Geometry: see drawing. Coordinates: mm, zero at the bounding-box minimum. A direction names the side the tool comes from. Coordinates: 2 decimals unless noted, no trailing zeros. Write each loop counter-clockwise with the first axis right and the second up, starting at its lowest first coordinate (ties: lowest second). Pieces come first, ordered by that corner, then holes.
1) Section query A-A (x = 18.85). Output: boundary loops of the cut face in (y, z), then the cut area to 3 significant figures.
2) Section query D-D (z = 5). Output: boundary loops of the cut face in (x, y).
3) Set-up query: the marked faces 1 and 2. Return all of +Z, -Z, +X, -X, +Y, -Y with unobstructed straight access to the full face (end or side cutting, diameter ignored); none if empty.
4) Section query B-B (z = 24.09). Output: boundary loops of the cut face in (x, y), then the cut area to 3 significant figures.
5) Section query C-C (x = 29.85). Output: boundary loops of the cut face in (y, z).
6) Line query: L1, parallel to Y at x = 5, z = 24.09; L2, parallel to Y at x = 29.85, z = 8.3; L3, parallel to Y at x = 40.85, z = 5.5. Output: solid intervals per line, ascending.
7) Pin query (flat end, axial travel): pin 1 Ø4 at (y, z) = (10, 49.09) entering from +X; pin 2 Ø16.5 at (x, y) = (29.85, 20) entering from +Z; pin 3 Ø1 at (x, y) = (43.5, 29.5) entering from +Z. Return the tip coordinate at first contact, or that it passes through.
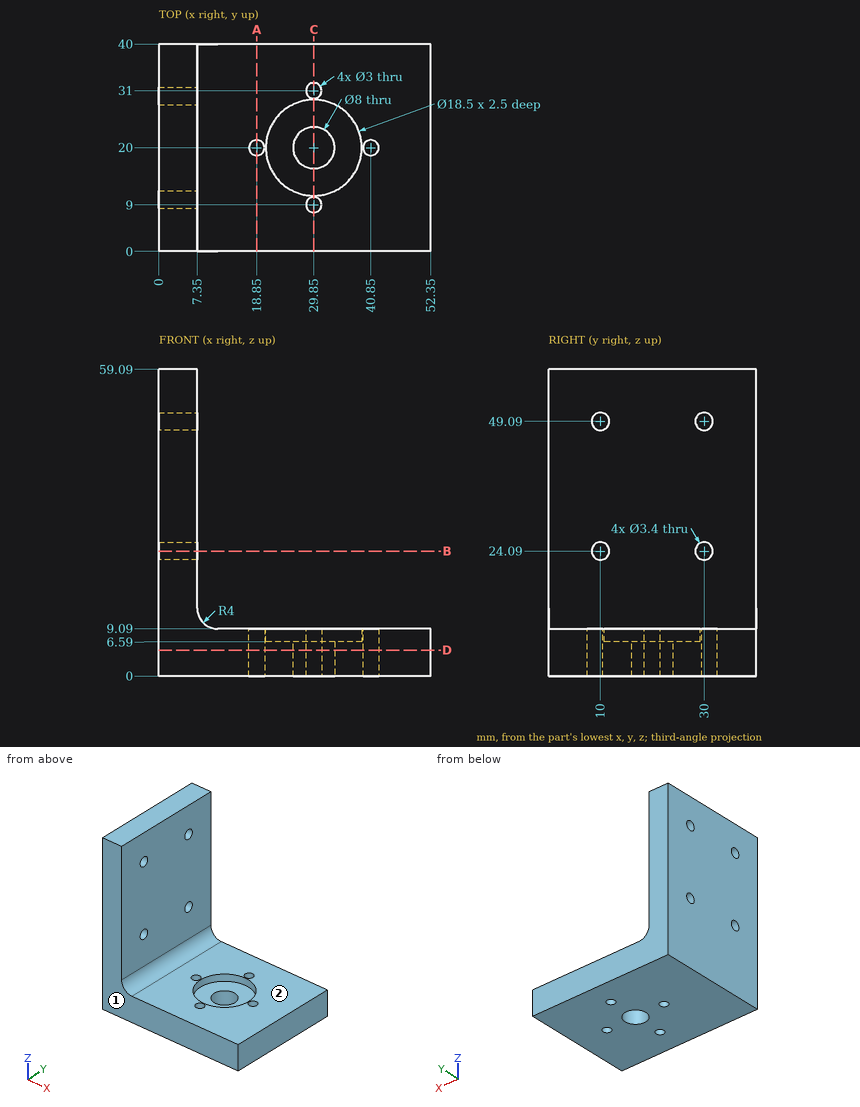
Answer:
1. outline: (0, 0) - (18.5, 0) - (18.5, 9.09) - (0, 9.09) - close; (21.5, 0) - (40, 0) - (40, 9.09) - (21.5, 9.09) - close
1. area: 336 mm2
2. outline: (0, 0) - (52.35, 0) - (52.35, 40) - (0, 40) - close; hole circle Ø3 at (18.85, 20); hole circle Ø8 at (29.85, 20); hole circle Ø3 at (29.85, 9); hole circle Ø3 at (29.85, 31); hole circle Ø3 at (40.85, 20)
3. face 1: +Z, -Z, +X, -X, -Y
3. face 2: +Z, +X, +Y, -Y
4. outline: (0, 0) - (7.35, 0) - (7.35, 8.3) - (0, 8.3) - close; (0, 11.7) - (7.35, 11.7) - (7.35, 28.3) - (0, 28.3) - close; (0, 31.7) - (7.35, 31.7) - (7.35, 40) - (0, 40) - close
4. area: 244 mm2
5. outline: (0, 0) - (7.5, 0) - (7.5, 9.09) - (0, 9.09) - close; (10.5, 0) - (16, 0) - (16, 6.59) - (10.75, 6.59) - (10.75, 9.09) - (10.5, 9.09) - close; (24, 0) - (29.5, 0) - (29.5, 9.09) - (29.25, 9.09) - (29.25, 6.59) - (24, 6.59) - close; (32.5, 0) - (40, 0) - (40, 9.09) - (32.5, 9.09) - close
6. L1: y = 0 to 8.3, 11.7 to 28.3, 31.7 to 40
6. L2: y = 0 to 7.5, 10.5 to 10.75, 29.25 to 29.5, 32.5 to 40
6. L3: y = 0 to 18.5, 21.5 to 40
7. pin 1: stops at x = 7.35
7. pin 2: stops at z = 6.59
7. pin 3: stops at z = 9.09
